Source: three-view drawing plus pictorial views. Frame: mm from the lowest corner of the part. Round coordinates to 2 decimals unless told otherwise and drop trailing zeros. Loops run counter-clockwise (first coordinate to the right, second up) from the corner with the lowest first, then second, coordinate; pieces in that order, holes last. Notation, with made-up numbers: M -17.75,-4 L 5.25,-4 A26 cw 5.25,25 Z; hole C -15,-10 d3. An arc over 180 degrees is marked long. Return JSON: item names as keys, results as strings. Group by question number.
1) Material intervals for line 1 (Y direction, x = 40.5, z = 0.8); line 2 (Y direction, x = 38.5, z = 0.95); line 3 (X direction, y = 58.5, z = 0.8), sorted ascending. Write a range as from..to.
2) Section D-D (y = 37.5). Output: boundary loops of the cut face in (x, z), plus the area to 3 significant figures.
3) Section A-A (x = 10). Output: boundary loops of the cut face in (y, z).
4) Section C-C (z = 1.3). Output: boundary loops of the cut face in (x, y).
5) Section B-B (y = 30). Output: boundary loops of the cut face in (x, z), plus the area to 3 significant figures.
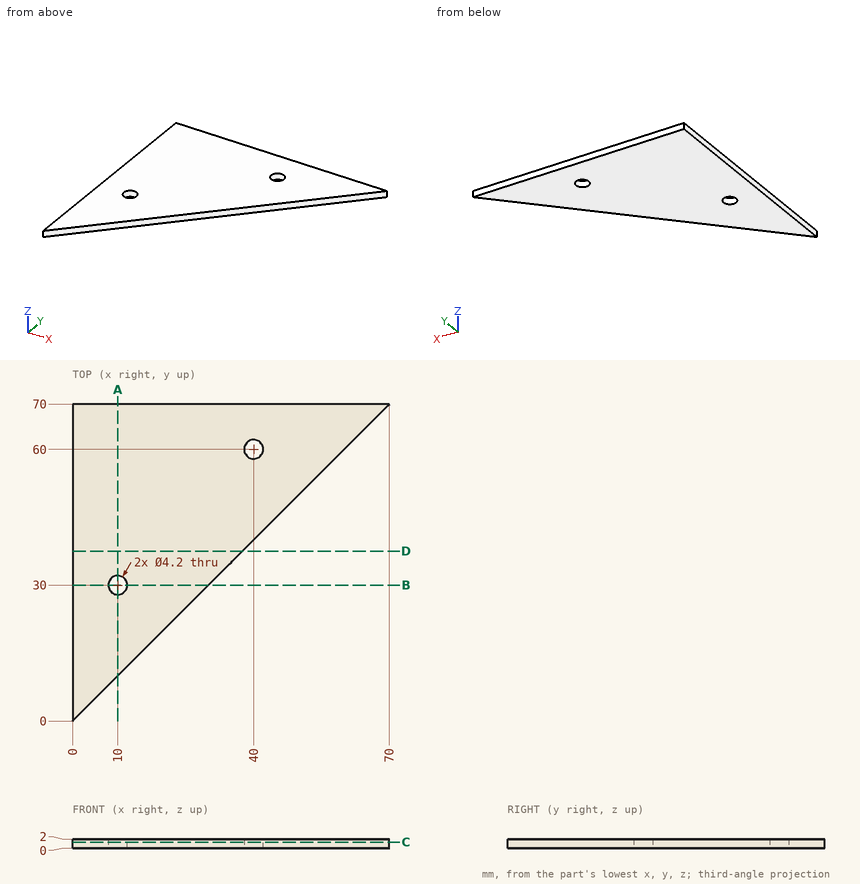
Returned:
{
 "1": {"line 1": "y = 40.5..57.96, 62.04..70", "line 2": "y = 38.5..58.53, 61.47..70", "line 3": "x = 0..38.53, 41.47..58.5"},
 "2": {"outline": "M 0,0 L 37.5,0 L 37.5,2 L 0,2 Z", "area": "75.0 mm^2"},
 "3": {"outline": "M 10,0 L 27.9,0 L 27.9,2 L 10,2 Z; M 32.1,0 L 70,0 L 70,2 L 32.1,2 Z"},
 "4": {"outline": "M 0,0 L 70,70 L 0,70 Z; hole C 10,30 d4.2; hole C 40,60 d4.2"},
 "5": {"outline": "M 0,0 L 7.9,0 L 7.9,2 L 0,2 Z; M 12.1,0 L 30,0 L 30,2 L 12.1,2 Z", "area": "51.6 mm^2"}
}
